```python
from build123d import *

# Parameters (mm, degrees)
EXTRUDE_3344_DEPTH     = 10
EXTRUDE_7001_DEPTH     = 10
CUT_EXTRUDE_7885_REACH = 1081.252
SKETCH6_R              = 1.5
SKETCH10_R             = 4
CUT_EXTRUDE2_DEPTH     = 10


with BuildPart() as part:
    # Sketch 366 → Extrude 3344 (new body)
    with BuildSketch(Plane.XY):
        with BuildLine():
            Line((398.785011417, -200.651493516), (-79.294784876, -202.700029576))
            add(Edge.make_bspline(
                [(-79.294784876, -202.700029576), (-78.517207033, -227.700030074), (-66.77413567, -249.709423293), (-44.177194857, -268.758733778)],
                knots=[0.130434783, 0.130434783, 0.130434783, 0.130434783, 0.173913043, 0.173913043, 0.173913043, 0.173913043], degree=3))
            add(Edge.make_bspline(
                [(-44.177194857, -268.758733778), (-12.705791537, -245.829015584), (38.959692419, -231.734357298), (82.666649693, -241.803965427)],
                knots=[0.173913043, 0.173913043, 0.173913043, 0.173913043, 0.217391304, 0.217391304, 0.217391304, 0.217391304], degree=3))
            add(Edge.make_bspline(
                [(82.666649693, -241.803965427), (105.678664452, -251.652519997), (111.246401119, -268.691898993), (94.211511027, -290.72343747)],
                knots=[0.217391304, 0.217391304, 0.217391304, 0.217391304, 0.260869565, 0.260869565, 0.260869565, 0.260869565], degree=3))
            add(Edge.make_bspline(
                [(94.211511027, -290.72343747), (87.158146802, -299.84568745), (74.983143168, -308.421687748), (61.059861243, -320.502125148)],
                knots=[0.260869565, 0.260869565, 0.260869565, 0.260869565, 0.304347826, 0.304347826, 0.304347826, 0.304347826], degree=3))
            add(Edge.make_bspline(
                [(61.059861243, -320.502125148), (47.380576162, -331.841195194), (34.883169502, -345.267804883), (22.870464668, -359.106695422)],
                knots=[0.304347826, 0.304347826, 0.304347826, 0.304347826, 0.347826087, 0.347826087, 0.347826087, 0.347826087], degree=3))
            add(Edge.make_bspline(
                [(22.870464668, -359.106695422), (-5.584395486, -391.889656597), (-25.592236503, -386.636342684), (-46.417157713, -376.787588607)],
                knots=[0.347826087, 0.347826087, 0.347826087, 0.347826087, 0.391304348, 0.391304348, 0.391304348, 0.391304348], degree=3))
            add(Edge.make_bspline(
                [(-46.417157713, -376.787588607), (-71.990241561, -366.221906762), (-92.784039707, -356.68149048), (-112.974728727, -345.609360564)],
                knots=[0.391304348, 0.391304348, 0.391304348, 0.391304348, 0.434782609, 0.434782609, 0.434782609, 0.434782609], degree=3))
            ThreePointArc((-112.974728727, -345.609360564), (-147.291018167, -331.50605668), (-183.878601839, -325.353039337))
            ThreePointArc((-183.878601839, -325.353039337), (-234.41691777, -376.347060605), (-177.788935429, -420.480757462))
            ThreePointArc((-177.788935429, -420.480757462), (-128.557787466, -442.172804122), (-130.703269603, -495.928247794))
            ThreePointArc((-130.703269603, -495.928247794), (-178.505297895, -598.929354982), (-181.694355183, -712.437468808))
            add(Edge.make_bspline(
                [(-181.694355183, -712.437468808), (138.462224148, -807.731703363), (410.691079854, -765.39904884), (650.190442214, -612.598169561)],
                knots=[0.652173913, 0.652173913, 0.652173913, 0.652173913, 0.695652174, 0.695652174, 0.695652174, 0.695652174], degree=3))
            add(Edge.make_bspline(
                [(650.190442214, -612.598169561), (721.726306985, -555.13661338), (771.374178439, -572.802842814), (761.971022851, -542.438303349)],
                knots=[0.695652174, 0.695652174, 0.695652174, 0.695652174, 0.739130435, 0.739130435, 0.739130435, 0.739130435], degree=3))
            add(Edge.make_bspline(
                [(761.971022851, -542.438303349), (749.988144288, -518.251093648), (723.103402832, -500.836242812), (635.239899657, -505.006434182)],
                knots=[0.739130435, 0.739130435, 0.739130435, 0.739130435, 0.782608696, 0.782608696, 0.782608696, 0.782608696], degree=3))
            add(Edge.make_bspline(
                [(635.239899657, -505.006434182), (572.991975282, -501.932832065), (433.550272387, -486.778792548), (380.910397107, -452.903731023)],
                knots=[0.782608696, 0.782608696, 0.782608696, 0.782608696, 0.826086957, 0.826086957, 0.826086957, 0.826086957], degree=3))
            add(Edge.make_bspline(
                [(380.910397107, -452.903731023), (364.765905966, -442.514313456), (356.786231562, -430.363849161), (361.702578451, -416.260911342)],
                knots=[0.826086957, 0.826086957, 0.826086957, 0.826086957, 0.869565217, 0.869565217, 0.869565217, 0.869565217], degree=3))
            add(Edge.make_bspline(
                [(361.702578451, -416.260911342), (369.757666434, -319.561849491), (455.747401527, -287.137003064), (480.242749516, -200.302456329)],
                knots=[0.869565217, 0.869565217, 0.869565217, 0.869565217, 0.913043478, 0.913043478, 0.913043478, 0.913043478], degree=3))
            add(Edge.make_bspline(
                [(480.242749516, -200.302456329), (553.544349425, -5.601453319), (495.010045056, 115.276837959), (568.085803242, 187.174308847)],
                knots=[0.913043478, 0.913043478, 0.913043478, 0.913043478, 0.956521739, 0.956521739, 0.956521739, 0.956521739], degree=3))
            ThreePointArc((568.085803242, 187.174308847), (593.606841589, 203.592061702), (604.925253944, 231.748047725))
            ThreePointArc((604.925253944, 231.748047725), (600.64196866, 247.878688747), (587.30163028, 257.907621119))
            ThreePointArc((587.30163028, 257.907621119), (571.737485415, 260.097118561), (556.344046154, 256.922448156))
            add(Edge.make_bspline(
                [(556.344046154, 256.922448156), (413.493143177, 200.699964154), (492.80385804, -30.446360595), (410.726691822, -175.599321984)],
                knots=[0.000400641, 0.000400641, 0.000400641, 0.000400641, 0.043478261, 0.043478261, 0.043478261, 0.043478261], degree=3))
            add(Edge.make_bspline(
                [(410.726691822, -175.599321984), (407.231033021, -184.649150987), (403.219250068, -192.928185379), (398.785011417, -200.651493516)],
                knots=[0.043478261, 0.043478261, 0.043478261, 0.043478261, 0.086956522, 0.086956522, 0.086956522, 0.086956522], degree=3))
        make_face()
        with BuildLine():
            ThreePointArc((560.346734066, -608.221488629), (578.34219742, -573.494082411), (548.198906447, -548.569968521))
            ThreePointArc((548.198906447, -548.569968521), (285.319700334, -537.637629059), (23.550736383, -511.142298049))
            ThreePointArc((23.550736383, -511.142298049), (15.100477301, -511.443853236), (7.211162456, -514.486307076))
            ThreePointArc((7.211162456, -514.486307076), (-41.568101768, -557.565567627), (-70.986403303, -615.615570579))
            ThreePointArc((-70.986403303, -615.615570579), (-67.830334276, -649.354197638), (-42.606278131, -671.981674723))
            add(Edge.make_bspline(
                [(452.957398359, -655.370237863), (274.711219353, -724.494962923), (109.739326577, -728.980973594), (-42.606278131, -671.981674723)],
                knots=[0.555555556, 0.555555556, 0.555555556, 0.555555556, 0.666666667, 0.666666667, 0.666666667, 0.666666667], degree=3))
            add(Edge.make_bspline(
                [(560.346734066, -608.221488629), (524.550322081, -623.937738374), (490.70019891, -640.488126146), (452.957398359, -655.370237863)],
                knots=[0.444444444, 0.444444444, 0.444444444, 0.444444444, 0.555555556, 0.555555556, 0.555555556, 0.555555556], degree=3))
        make_face(mode=Mode.SUBTRACT)
        with BuildLine():
            add(Edge.make_bspline(
                [(97.461776435, -368.948566513), (168.620673064, -296.351125936), (255.441952596, -250.089184531), (374.508522413, -234.330838847)],
                knots=[0.75, 0.75, 0.75, 0.75, 1, 1, 1, 1], degree=3))
            add(Edge.make_bspline(
                [(374.508522413, -234.330838847), (336.704373514, -278.003480948), (285.636212987, -310.964302456), (247.882738821, -396.645799506)],
                knots=[0, 0, 0, 0, 0.25, 0.25, 0.25, 0.25], degree=3))
            add(Edge.make_bspline(
                [(247.882738821, -396.645799506), (222.475445143, -441.097914765), (152.691350033, -451.719558275), (92.090753497, -427.546413805)],
                knots=[0.25, 0.25, 0.25, 0.25, 0.5, 0.5, 0.5, 0.5], degree=3))
            add(Edge.make_bspline(
                [(92.090753497, -427.546413805), (69.794668972, -412.531131284), (70.490548771, -396.456667038), (97.461776435, -368.948566513)],
                knots=[0.5, 0.5, 0.5, 0.5, 0.75, 0.75, 0.75, 0.75], degree=3))
        make_face(mode=Mode.SUBTRACT)
    extrude(amount=EXTRUDE_3344_DEPTH)

    # Sketch5 → Extrude 7001 (add)
    with BuildSketch(Plane.XY.offset(10)):
        Polygon((40.661264648, -192.185935101), (90.66080564, -191.971690819), (90.703654496, -201.971599017), (40.704113505, -202.185843299), align=None)
        Polygon((240.659428615, -191.328957973), (290.658969607, -191.114713691), (290.701818463, -201.114621889), (240.702277472, -201.328866171), align=None)
    extrude(amount=-EXTRUDE_7001_DEPTH)

    # Sketch6 → Cut-Extrude 7885 (cut, up to next)
    with BuildSketch(Plane.XY.offset(10), mode=Mode.PRIVATE) as cut_extrude_7885_sk1:
        with Locations((531.551481114, -650.112952006)):
            Circle(SKETCH6_R)
    cut_extrude_7885_tool1 = extrude(cut_extrude_7885_sk1.sketch, amount=-CUT_EXTRUDE_7885_REACH, mode=Mode.PRIVATE) & part.part
    # Sketch6 → Cut-Extrude 7885 (cut, up to next)
    with BuildSketch(Plane.XY.offset(10), mode=Mode.PRIVATE) as cut_extrude_7885_sk2:
        with Locations((-118.7617531, -668.979567573)):
            Circle(SKETCH6_R)
    cut_extrude_7885_tool2 = extrude(cut_extrude_7885_sk2.sketch, amount=-CUT_EXTRUDE_7885_REACH, mode=Mode.PRIVATE) & part.part
    # Sketch6 → Cut-Extrude 7885 (cut, up to next)
    with BuildSketch(Plane.XY.offset(10), mode=Mode.PRIVATE) as cut_extrude_7885_sk3:
        Polygon((-139.846242547, -659.668589925), (-141.805292897, -669.474818645), (-127.095949816, -672.413394171), (-125.136899465, -662.60716545), align=None)
    cut_extrude_7885_tool3 = extrude(cut_extrude_7885_sk3.sketch, amount=-CUT_EXTRUDE_7885_REACH, mode=Mode.PRIVATE) & part.part
    # Sketch6 → Cut-Extrude 7885 (cut, up to next)
    with BuildSketch(Plane.XY.offset(10), mode=Mode.PRIVATE) as cut_extrude_7885_sk4:
        Polygon((-112.386606734, -675.351969696), (-110.427556384, -665.545740975), (-95.718213303, -668.4843165), (-97.677263653, -678.290545221), align=None)
    cut_extrude_7885_tool4 = extrude(cut_extrude_7885_sk4.sketch, amount=-CUT_EXTRUDE_7885_REACH, mode=Mode.PRIVATE) & part.part
    # Sketch6 → Cut-Extrude 7885 (cut, up to next)
    with BuildSketch(Plane.XY.offset(10), mode=Mode.PRIVATE) as cut_extrude_7885_sk5:
        Polygon((554.142933289, -645.543894263), (540.435760059, -651.635971254), (536.374375399, -642.497855768), (550.081548628, -636.405778777), align=None)
    cut_extrude_7885_tool5 = extrude(cut_extrude_7885_sk5.sketch, amount=-CUT_EXTRUDE_7885_REACH, mode=Mode.PRIVATE) & part.part
    # Sketch6 → Cut-Extrude 7885 (cut, up to next)
    with BuildSketch(Plane.XY.offset(10), mode=Mode.PRIVATE) as cut_extrude_7885_sk6:
        Polygon((522.667202169, -648.589932758), (508.96002894, -654.682009749), (513.021413601, -663.820125235), (526.72858683, -657.728048245), align=None)
    cut_extrude_7885_tool6 = extrude(cut_extrude_7885_sk6.sketch, amount=-CUT_EXTRUDE_7885_REACH, mode=Mode.PRIVATE) & part.part
    add(cut_extrude_7885_tool1.solids().sort_by_distance((531.551481, -650.112952, 10))[0], mode=Mode.SUBTRACT)
    add(cut_extrude_7885_tool2.solids().sort_by_distance((-118.761753, -668.979568, 10))[0], mode=Mode.SUBTRACT)
    add(cut_extrude_7885_tool3.solids().sort_by_distance((-133.471096, -666.040992, 10))[0], mode=Mode.SUBTRACT)
    add(cut_extrude_7885_tool4.solids().sort_by_distance((-104.05241, -671.918143, 10))[0], mode=Mode.SUBTRACT)
    add(cut_extrude_7885_tool5.solids().sort_by_distance((545.258654, -644.020875, 10))[0], mode=Mode.SUBTRACT)
    add(cut_extrude_7885_tool6.solids().sort_by_distance((517.844308, -656.205029, 10))[0], mode=Mode.SUBTRACT)

    # Sketch10 → Cut-Extrude2 (cut)
    with BuildSketch(Plane.XY.offset(10)):
        with Locations((-58.805785282, -483.725185308)):
            Circle(SKETCH10_R)
        with Locations((343.930985097, -492.062373655)):
            Circle(SKETCH10_R)
        with Locations((583.096913772, 215.46802458)):
            Circle(SKETCH10_R)
    extrude(amount=-CUT_EXTRUDE2_DEPTH, mode=Mode.SUBTRACT)


solid = part.part
```
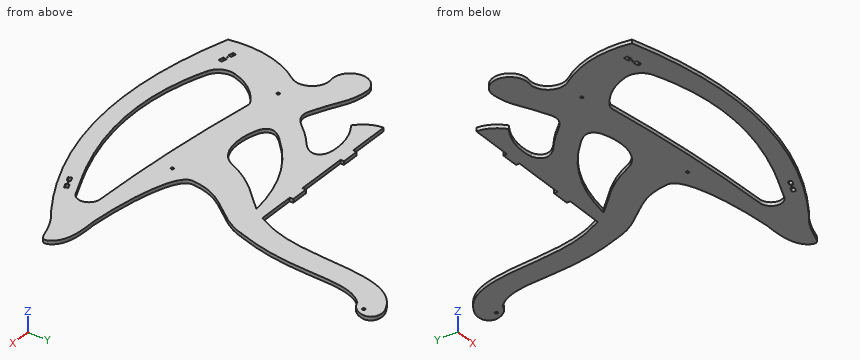
Verification items for the finished model (mm, model axes). Give positions to 0.01 mm unless a question says otherwise; leave off trailing zeros. Answer in a Markdown table with one row per item. Add a question column.
Item 1: Section check A-A, the plane x = 222. State how many separate pieces and enclosed holes the cut face has, and give its area (3 significant figures).
Item 2: Gauge pin test, flat ends, axial feed: pin 1 (2 mm diameter, centred on y = -520, z = 8, fed in from -X); pin 2 (2 mm diameter, centred on x = 486, z = 7, fed in from +Y); pin 3 (5 mm diameter, centred on y = -214.5, z = 4.5, fed in from +X). Record the tip position at first contact, or that the pin passes through.
Item 3: Scan lines: probe 1 along Y at (x, z) = (61.5, 6.5); probe 2 along Y at (x, z) = (66.5, 4); probe 3 along Y at (x, z) = (545.5, 3). Record each from-to range of solid material in increasing order. Write a range as from..to.
Filled sheet:
| question | item | result |
|---|---|---|
| 1 | separate pieces | 3 |
| 1 | enclosed holes | 0 |
| 1 | area | 2,370 mm^2 |
| 2 | pin 1 | stops at x = -147.28 |
| 2 | pin 2 | stops at y = 190.72 |
| 2 | pin 3 | stops at x = 476.47 |
| 3 | probe 1 | y = -759.58..-700.96, -515.96..-320.12, -238.78..-192.1 |
| 3 | probe 2 | y = -759.99..-701.87, -516.57..-315.87, -239.18..-192.08 |
| 3 | probe 3 | y = -671.24..-649.39, -638.44..-614.82, -548.54..-496.66, 156.24..252.11 |
